The figure shows three views and two pictorial views of one solid part (mm, origin at its lowest corner). Answer the questions. A direction names the side the tool comes from. Coordinates: 2 decimals unless noted, no trailing zeros. Order: outer loops, then holes, each group sorted by start corner. A loop starts at its lowest first (then second) coordinate and runs counter-clockwise, first axis right, second up. Notation, with made-up numbers: (-21, 51.5) - (23, 51.5) arc R18 cw to (23, 70.5) - close; hole circle Ø10 at (62, 37). An arc over 180 degrees is marked (long way). Use one line per item in the form item = value. Start each with the question number.
Item 1: The mould has two halves that part along Z. Classify the marked faces 3, 4 and 5: released by +Z, released by -Z, zero draft, split by the parting line, or undercut.
Item 2: A tool of negligible diameter and unlimited length cuts with its end or side. For the marked faces 1 and 2, from which of +Z, -Z, +X, -X, +Y, -Y can it reach the whole face along a straight path? Write none if from no direction.
Item 3: Section A-A, the plane x = 2.75 is taken. Write down the section's boundary in (y, z).
Item 4: Section B-B, the plane z = 2.1 is taken. Write down the section's boundary in (x, y).
Item 5: Section C-C, the plane y = 8.25 is taken. Write down the section's boundary in (x, z).
Item 6: Consider line 1 along Y through (x, z) = (2.1, 0.4); line 2 along Y through (x, z) = (2.8, 3); line 3 along Z through (x, y) = (2.6, 17.75). Determine where each line is inside the solid, lowest interval first. Write a range as [from, to].
Item 7: Section D-D, the plane z = 4.75 is taken. Write down the section's boundary in (x, y).
Item 8: Each of these flat-tipped pins is pushed along its axis until it touches: pin 1 Ø2 at (x, y) = (1, 11) entering from +Z; pin 2 Ø1.5 at (x, y) = (3.5, 21.5) entering from +Z; pin 3 Ø1.5 at (y, z) = (17, 1.5) entering from -X (1 decimal). Where does it stop, or does it pass through?
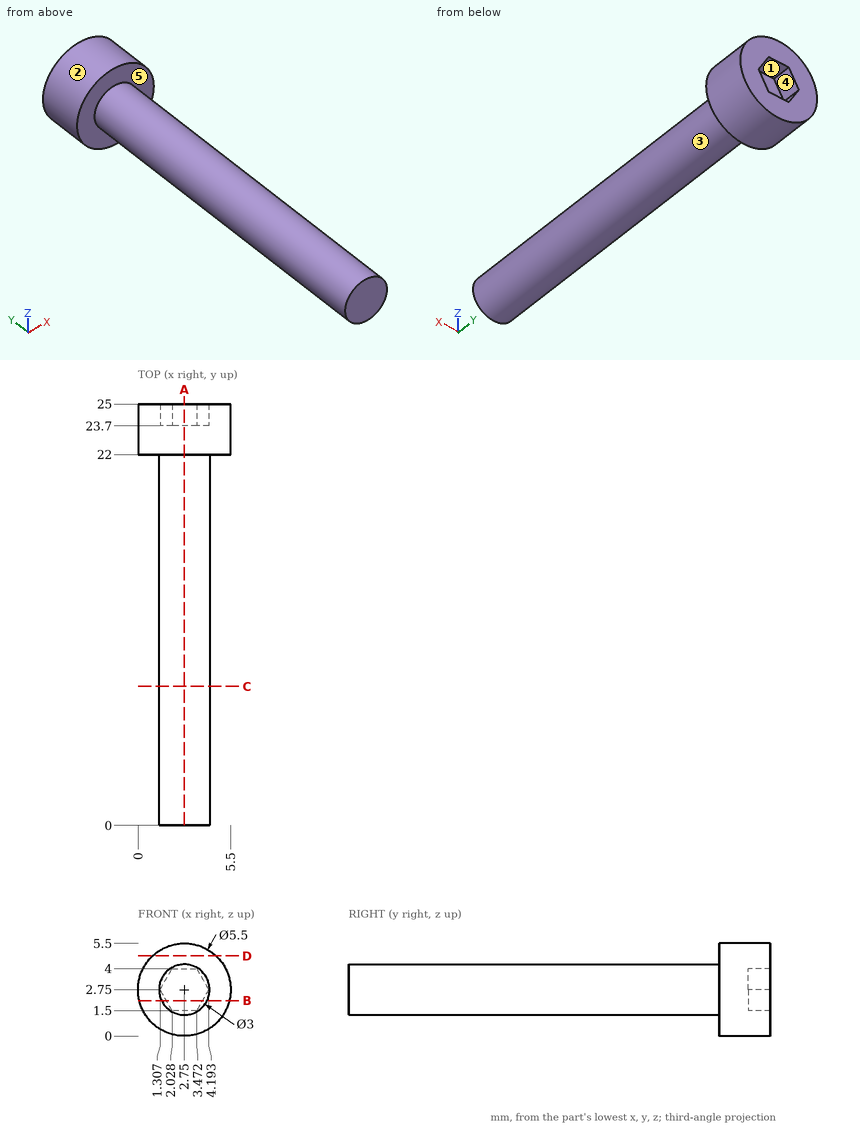
Response:
q1.face_3 = split by the parting line
q1.face_4 = undercut
q1.face_5 = zero draft
q2.face_1 = +Y
q2.face_2 = +Y, -Y
q3.outline = (0, 1.25) - (22, 1.25) - (22, 0) - (25, 0) - (25, 1.5) - (23.7, 1.5) - (23.7, 4) - (25, 4) - (25, 5.5) - (22, 5.5) - (22, 4.25) - (0, 4.25) - close
q4.outline = (0.08, 22) - (1.4, 22) - (1.4, 0) - (4.1, 0) - (4.1, 22) - (5.42, 22) - (5.42, 25) - (3.82, 25) - (3.82, 23.7) - (1.68, 23.7) - (1.68, 25) - (0.08, 25) - close
q5.outline = circle Ø3 at (2.75, 2.75)
q6.line_1 = [22, 25]
q6.line_2 = [0, 23.7]
q6.line_3 = [1.26, 4.24]
q7.outline = (0.86, 22) - (4.64, 22) - (4.64, 25) - (0.86, 25) - close
q8.pin_1 = 4.05
q8.pin_2 = 5.49
q8.pin_3 = 1.3
